Build history of the part. All positions in model axes, mm. Face numbers are marked on the shaded views. A direction names the side the tool comes from. Round coordinates to 2 decimals unless told otherwise and drop trailing zeros. Write each loop counter-clockwise with the first axis right and the second up, starting at its lowest first coordinate (ties: lowest second). Pieces come first, ordered by that corner, then holes. Notation, with made-up numbers: (51, 62) -> (80, 62) arc R19 cw to (80, 76) -> close; hole circle Ø10 at (-29, 5). An arc over 180 degrees is marked (long way). Answer in a Markdown table with one row per item. Add a question column.
from build123d import *

# Parameters (mm, degrees)
SKETCH1_R           = 2.1
BOSS_EXTRUDE2_DEPTH = 17
SKETCH4_R           = 4.5
BOSS_EXTRUDE3_DEPTH = 1.5
SKETCH5_R           = 2.5
BOSS_EXTRUDE4_DEPTH = 2
SKETCH8_R           = 2.1
CUT_EXTRUDE1_DEPTH  = 16.2
BOSS_EXTRUDE6_DEPTH = 6.2


with BuildPart() as part:
    # Sketch1 → Boss-Extrude2 (new body)
    with BuildSketch(Plane(origin=(0, 0, 0), x_dir=(1, 0, 0), z_dir=(0, 1, 0))):
        with BuildLine():
            Line((-8.5, -20), (8.5, -20))
            Line((8.5, -20), (8.5, -15.297058541))
            ThreePointArc((8.5, -15.297058541), (16.311372932, -6.339488392), (16.599242405, 5.542125186))
            Line((16.599242405, 5.542125186), (19.936533479, 7.468911087))
            ThreePointArc((19.936533479, 7.468911087), (21.217622393, 12.25), (16.436533479, 13.531088913))
            Line((16.436533479, 13.531088913), (13.099242405, 11.604303013))
            ThreePointArc((13.099242405, 11.604303013), (-8.75, 15.155444566), (-16.599242405, -5.542125186))
            Line((-16.599242405, -5.542125186), (-19.936533479, -7.468911087))
            ThreePointArc((-19.936533479, -7.468911087), (-21.217622393, -12.25), (-16.436533479, -13.531088913))
            Line((-16.436533479, -13.531088913), (-13.099242405, -11.604303013))
            ThreePointArc((-13.099242405, -11.604303013), (-10.956319134, -13.64584446), (-8.5, -15.297058541))
            Line((-8.5, -15.297058541), (-8.5, -20))
        make_face()
        with Locations((-18.186533479, -10.5)):
            Circle(SKETCH1_R, mode=Mode.SUBTRACT)
        with Locations((18.186533479, 10.5)):
            Circle(SKETCH1_R, mode=Mode.SUBTRACT)
    extrude(amount=BOSS_EXTRUDE2_DEPTH)

    # Sketch4 → Boss-Extrude3 (add)
    with BuildSketch(Plane(origin=(0, 17, 0), x_dir=(1, 0, 0), z_dir=(0, 1, 0))):
        with Locations((-5, 8.660254038)):
            Circle(SKETCH4_R)
    extrude(amount=BOSS_EXTRUDE3_DEPTH)

    # Sketch5 → Boss-Extrude4 (add)
    with BuildSketch(Plane(origin=(0, 18.5, 0), x_dir=(1, 0, 0), z_dir=(0, 1, 0))):
        with Locations((-5, 8.660254038)):
            Circle(SKETCH5_R)
    extrude(amount=BOSS_EXTRUDE4_DEPTH)

    # Sketch8 → Cut-Extrude1 (cut)
    with BuildSketch(Plane.XZ):
        with BuildLine():
            ThreePointArc((16.599242405, -5.542125186), (15.155444566, -8.75), (13.099242405, -11.604303013))
            Line((13.099242405, -11.604303013), (16.436533479, -13.531088913))
            ThreePointArc((16.436533479, -13.531088913), (21.217622393, -12.25), (19.936533479, -7.468911087))
            Line((19.936533479, -7.468911087), (16.599242405, -5.542125186))
        make_face()
        with Locations((18.186533479, -10.5)):
            Circle(SKETCH8_R, mode=Mode.SUBTRACT)
        with BuildLine():
            ThreePointArc((-13.099242405, 11.604303013), (-15.155444566, 8.75), (-16.599242405, 5.542125186))
            Line((-16.599242405, 5.542125186), (-19.936533479, 7.468911087))
            ThreePointArc((-19.936533479, 7.468911087), (-21.217622393, 12.25), (-16.436533479, 13.531088913))
            Line((-16.436533479, 13.531088913), (-13.099242405, 11.604303013))
        make_face()
        with Locations((-18.186533479, 10.5)):
            Circle(SKETCH8_R, mode=Mode.SUBTRACT)
    extrude(amount=-CUT_EXTRUDE1_DEPTH, mode=Mode.SUBTRACT)

    # Sketch9 → Boss-Extrude6 (add)
    with BuildSketch(Plane(origin=(0, 20.5, 0), x_dir=(1, 0, 0), z_dir=(0, 1, 0))):
        with BuildLine():
            Line((-7, 7.160254038), (-3, 7.160254038))
            ThreePointArc((-3, 7.160254038), (-2.5, 8.660254038), (-3, 10.160254038))
            Line((-3, 10.160254038), (-7, 10.160254038))
            ThreePointArc((-7, 10.160254038), (-7.5, 8.660254038), (-7, 7.160254038))
        make_face()
    extrude(amount=BOSS_EXTRUDE6_DEPTH)


solid = part.part
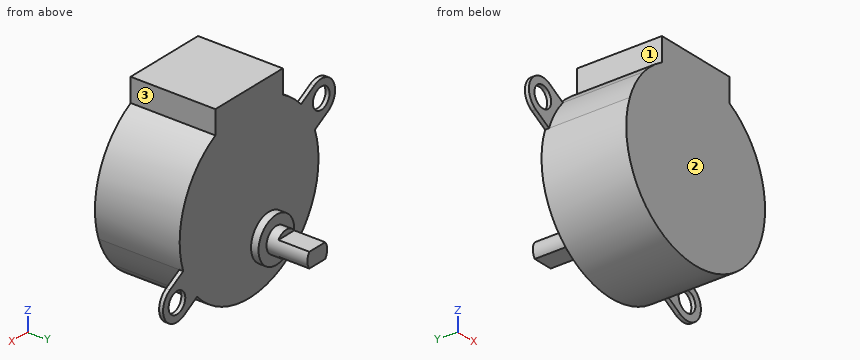
(1) Probe line 1 along Y through (x, z) = (7, 5); line 2 along X through (y, z) = (16.8, -10.5); line 3 along X through (y, z) = (5.25, -10.5). List the from-to ranges inside material, lowest first.
(2) Saw through at B-B (y = 3.75). List the corners of the cut face in (x, z).
(3) Drop flat-ended pins along their axis: P1, Ø1.4, axis at y = 12.5, z = 18, coming from the +X side; P2, Ø6, axis at y = 11.5, z = 1, coming from the -X side; P3, Ø12, axis at y = 5.5, z = -7, coming from the +X side. Give the stop position or say it passes through.
(4) Which spindle directions (+Z, -Z, +X, -X, +Y, -Y) get a long thin tool onto all of the face, cutting with end or side? Do the marked faces 1, 2 and 3. Say none if no direction does.
(5) Saw through at A-A (z = 10.5). List the corners of the cut face in (x, y), plus the area to 3 significant figures.
(6) Saw through at D-D (z = 0). List the corners of the cut face in (x, y).
(7) Saw through at C-C (x = -5). List the corners of the cut face in (y, z).
Answer sheet:
| question | item | result |
|---|---|---|
| 1 | line 1 | y = 0 to 17 |
| 1 | line 2 | x = -14 to 16.09, 20.29 to 21.69 |
| 1 | line 3 | x = -14 to 14 |
| 2 | outline | (-8.5, 15.3) arc R17.5 ccw (long way) to (8.5, 15.3) -> (8.5, 20) -> (-8.5, 20) -> close |
| 3 | P1 | stops at x = 8.5 |
| 3 | P2 | stops at x = -17.5 |
| 3 | P3 | stops at x = 17.47 |
| 4 | face 1 | +Z, -X, +Y, -Y |
| 4 | face 2 | +Z, -Z, +X, -X, -Y |
| 4 | face 3 | +Z, +X, +Y, -Y |
| 5 | outline | (-21.69, 16.2) -> (-20.29, 16.2) -> (-20.29, 17) -> (-21.69, 17) -> close; (-16.09, 16.2) -> (-14, 16.2) -> (-14, 0) -> (14, 0) -> (14, 17) -> (-16.09, 17) -> close |
| 5 | area | 479 mm² |
| 6 | outline | (-17.5, 0) -> (17.5, 0) -> (17.5, 17) -> (-17.5, 17) -> close |
| 7 | outline | (0, -16.77) -> (17, -16.77) -> (17, -13.16) -> (18.5, -13.16) -> (18.5, -11.16) -> (20.5, -11.16) -> (20.5, -10.16) -> (26.7, -10.16) -> (26.7, -7.16) -> (20.5, -7.16) -> (20.5, -6.16) -> (18.5, -6.16) -> (18.5, -4.16) -> (17, -4.16) -> (17, 20) -> (0, 20) -> close |
